The model under review builds one solid part; all positions refer to its coordinate system, in mm. Give positions to 0.01 mm unless a question says otherwise; leave off trailing zeros. Loops run counter-clockwise (first coordinate to the right, second up) from the corner with the lowest first, then second, coordinate; pieces in that order, holes last. Notation, with made-up numbers: M 25.25,-31.5 L 59.25,-31.5 A24 ccw 59.25,2.5 Z; hole C 82,-38.5 d9. An arc over 180 degrees is marked long. One line per item, written item: value. Start each with the question number.
Q1. For pin 1 (8 mm diameter, centred on x = 1, z = -183.5, fed in from +Y); pin 2 (8 mm diameter, centred on x = 1.5, z = -140.5, fed in from +Y); pin 3 (1 mm diameter, centred on y = -1, z = -61, fed in from +X), all flat-tipped, find the tip position at first contact; note any pin that passes through.
Q2. We need section A-A on y = -1.75. Write out the cut boundary in (x, z), plus the area to 3 significant figures.
Q3. To check wall thickness, follow line 1 along Y through (x, z) = (7, -114.5); line 2 along X through (y, z) = (9.75, -235); line 3 along X through (y, z) = (-10.5, -126). State the ranges of each line that lie inside material, in increasing order. Write a range as from..to.
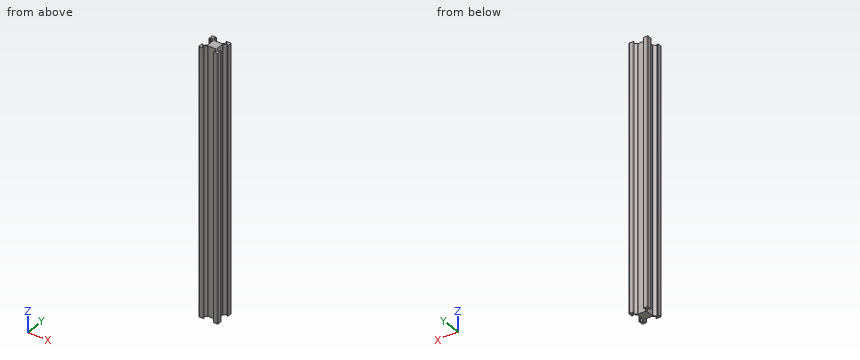
```python
from build123d import *

# Parameters (mm, degrees)
BOSS_EXTRUDE1_DEPTH = 355.6
FILLET1_R           = 0.79375


with BuildPart() as part:
    # Sketch1 → Boss-Extrude1 (new body)
    with BuildSketch(Plane.XY):
        Polygon((-6.35, -5.227467985), (-6.35, 5.227467985), (-11.1125, 9.989967985), (-11.1125, 6.35), (-12.7, 6.35), (-12.7, 12.7), (-6.35, 12.7), (-6.35, 11.1125), (-9.989967985, 11.1125), (-5.227467985, 6.35), (5.227467985, 6.35), (9.989967985, 11.1125), (6.35, 11.1125), (6.35, 12.7), (12.7, 12.7), (12.7, 6.35), (11.1125, 6.35), (11.1125, 9.989967985), (6.35, 5.227467985), (6.35, -5.227467985), (11.1125, -9.989967985), (11.1125, -6.35), (12.7, -6.35), (12.7, -12.7), (6.35, -12.7), (6.35, -11.1125), (9.989967985, -11.1125), (5.227467985, -6.35), (-5.227467985, -6.35), (-9.989967985, -11.1125), (-6.35, -11.1125), (-6.35, -12.7), (-12.7, -12.7), (-12.7, -6.35), (-11.1125, -6.35), (-11.1125, -9.989967985), align=None)
    extrude(amount=-BOSS_EXTRUDE1_DEPTH)

    # Fillet1
    fillet1_edges = [part.edges().sort_by_distance(p)[0] for p in [
        (-6.35, -11.1125, -177.8),
        (-6.35, -12.7, -177.8),
        (-12.7, -12.7, -177.8),
        (-12.7, -6.35, -177.8),
        (-11.1125, -6.35, -177.8),
        (-11.1125, -9.989967985, -177.8),
        (-6.35, -5.227467985, -177.8),
        (-6.35, 5.227467985, -177.8),
        (-11.1125, 9.989967985, -177.8),
        (-11.1125, 6.35, -177.8),
        (-12.7, 6.35, -177.8),
        (-12.7, 12.7, -177.8),
        (-6.35, 12.7, -177.8),
        (-6.35, 11.1125, -177.8),
        (-9.989967985, 11.1125, -177.8),
        (-5.227467985, 6.35, -177.8),
        (5.227467985, 6.35, -177.8),
        (9.989967985, 11.1125, -177.8),
        (6.35, 11.1125, -177.8),
        (6.35, 12.7, -177.8),
        (12.7, 12.7, -177.8),
        (12.7, 6.35, -177.8),
        (11.1125, 6.35, -177.8),
        (11.1125, 9.989967985, -177.8),
        (6.35, 5.227467985, -177.8),
        (6.35, -5.227467985, -177.8),
        (11.1125, -9.989967985, -177.8),
        (11.1125, -6.35, -177.8),
        (12.7, -6.35, -177.8),
        (12.7, -12.7, -177.8),
        (6.35, -12.7, -177.8),
        (6.35, -11.1125, -177.8),
        (9.989967985, -11.1125, -177.8),
        (5.227467985, -6.35, -177.8),
        (-5.227467985, -6.35, -177.8),
        (-9.989967985, -11.1125, -177.8),
    ]]
    fillet(fillet1_edges, radius=FILLET1_R - 0.0001)  # a hair under: the kernel refuses the full size


solid = part.part
```
Solved:
1. pin 1: y = 6.36
1. pin 2: y = 6.62
1. pin 3: x = 6.35
2. outline: M -6.35,-355.6 L 6.35,-355.6 L 6.35,0 L -6.35,0 Z
2. area: 4,520 mm2
3. line 1: -12.69..-11.13, -8.12..-5.88, 5.88..8.12, 11.13..12.69
3. line 2: -12.7..-8.63, 8.63..12.7
3. line 3: -12.7..-8.85, 8.85..12.7
